Can you work these out from the drawing? Everything is in mm from the part's minimum corner. A direction names the side the tool comes from. Round coordinates to 2 decimals unless told otherwise and drop trailing zeros. Loops run counter-clockwise (first coordinate to the right, second up) from the corner with the lowest first, then second, coordinate; pieces in that order, holes last. Notation, with made-up numbers: M 0,80.25 L 8,80.25 A20 ccw 8,92.25 Z; hole C -4.5,67 d5. An arc over 180 degrees is marked long. Use a Markdown table: item, result.
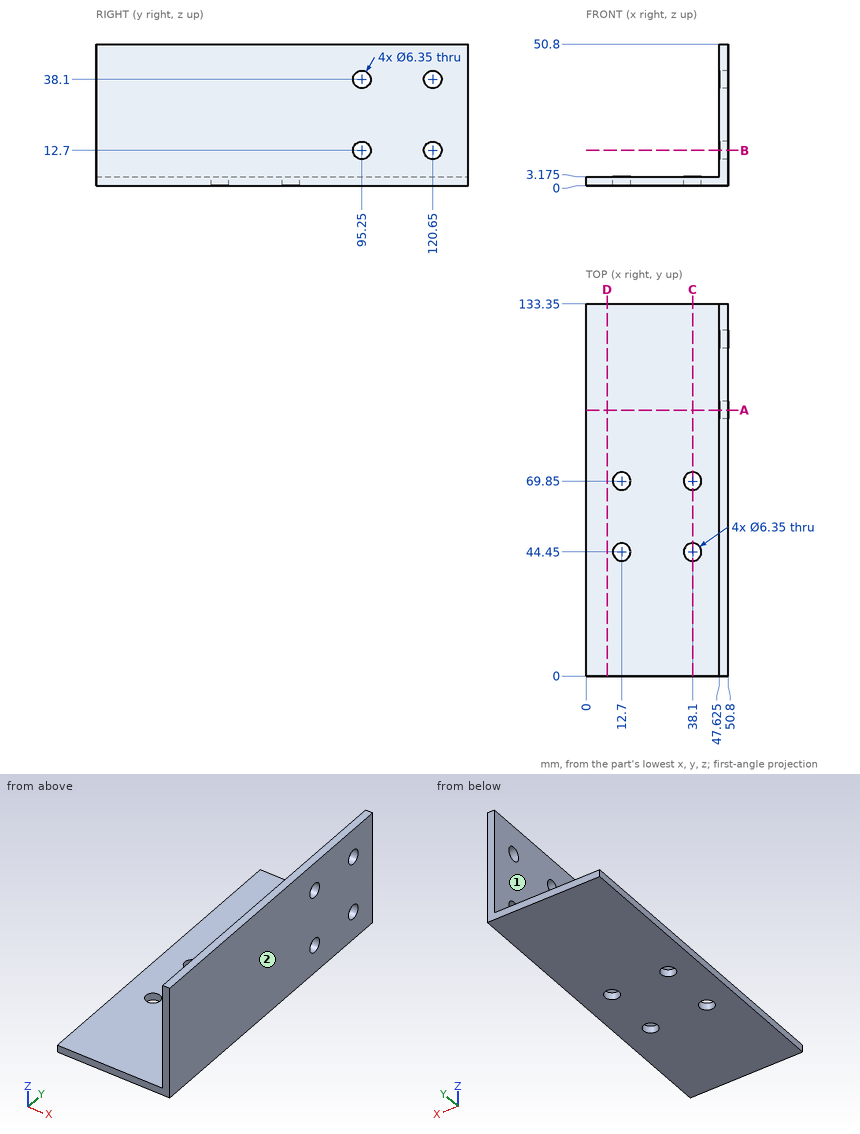
Q1. Imagine slicing it at A-A, the plane y = 95.25. Please give me the cut outline in (x, z) (3 decimals).
Return value:
| item | result |
|---|---|
| outline | M 0,0 L 50.8,0 L 50.8,9.525 L 47.625,9.525 L 47.625,3.175 L 0,3.175 Z; M 47.625,15.875 L 50.8,15.875 L 50.8,34.925 L 47.625,34.925 Z; M 47.625,41.275 L 50.8,41.275 L 50.8,50.8 L 47.625,50.8 Z |
Q2. Imagine slicing it at D-D, the plane x = 7.5. Please give me the cut outline in (y, z) (3 decimals), then the cut area to 3 significant figures.
Return value:
| item | result |
|---|---|
| outline | M 0,0 L 133.35,0 L 133.35,3.175 L 0,3.175 Z |
| area | 423 mm^2 |
Q3. Will these pins go through, and if not, where does the flat tip stop? P1, Ø10, axis at y = 53, z = 20, coming from the -X side (3 decimals); P2, Ø8.5, axis at x = 38.1, y = 69.85, coming from the -Z side; P3, Ø6, axis at x = 20.5, y = 117, coming from the +Z side (3 decimals); P4, Ø5.5, axis at y = 95.25, z = 12.7, coming from the +X side.
Return value:
| item | result |
|---|---|
| P1 | stops at x = 47.625 |
| P2 | stops at z = 0 |
| P3 | stops at z = 3.175 |
| P4 | passes through |
Q4. I need wall thicknesses on line 1 (X direction, y = 69.85, z = 1.25) (3 decimals); line 2 (Y direction, x = 38, z = 1). Which ranges of each line are inside material? Lowest first, please. Write a range as from..to.
Return value:
| item | result |
|---|---|
| line 1 | x = 0..9.525, 15.875..34.925, 41.275..50.8 |
| line 2 | y = 0..41.28, 47.62..66.68, 73.02..133.35 |
Q5. Imagine slicing it at B-B, the plane z = 12.7. Please give me the cut outline in (x, y) (3 decimals).
Return value:
| item | result |
|---|---|
| outline | M 47.625,0 L 50.8,0 L 50.8,92.075 L 47.625,92.075 Z; M 47.625,98.425 L 50.8,98.425 L 50.8,117.475 L 47.625,117.475 Z; M 47.625,123.825 L 50.8,123.825 L 50.8,133.35 L 47.625,133.35 Z |
Q6. For the marked faces 1 and 2, which set-ups out of +Z, -Z, +X, -X, +Y, -Y let a thin tool reach every point of the face, with its end or its side?
Return value:
| item | result |
|---|---|
| face 1 | +Z, -X, +Y, -Y |
| face 2 | +Z, -Z, +X, +Y, -Y |
Q7. Imagine slicing it at C-C, the plane x = 38.1. Please give me the cut outline in (y, z) (3 decimals).
Return value:
| item | result |
|---|---|
| outline | M 0,0 L 41.275,0 L 41.275,3.175 L 0,3.175 Z; M 47.625,0 L 66.675,0 L 66.675,3.175 L 47.625,3.175 Z; M 73.025,0 L 133.35,0 L 133.35,3.175 L 73.025,3.175 Z |
